```python
from build123d import *

# Parameters (mm, degrees)
SM_BASE_FLANGE_1_DEPTH = 90
CUT_EXTRUDE_1_DEPTH    = 10
CUT_EXTRUDE_2_DEPTH    = 10
FILLET_1_R             = 10


# Sheet-metal steps are written as plain solids
with BuildPart() as part:
    # Sketch 1 → 基体-法兰1 (new body)
    with BuildSketch(Plane.XY):
        with BuildLine():
            Line((0, 0), (34.731899525, 0))
            ThreePointArc((34.731899525, 0), (34.983831563, 0.044422416), (35.205376879, 0.172331663))
            Line((35.205376879, 0.172331663), (57.981333294, 19.283628291))
            Line((57.981333294, 19.283628291), (58.945514708, 18.134561626))
            Line((58.945514708, 18.134561626), (36.169558293, -0.976735001))
            ThreePointArc((36.169558293, -0.976735001), (35.496861778, -1.365116516), (34.731899525, -1.5))
            Line((34.731899525, -1.5), (0, -1.5))
            Line((0, -1.5), (0, 0))
        make_face()
    extrude(amount=SM_BASE_FLANGE_1_DEPTH)

    # 草图6 → 切除-拉伸1 (cut)
    with BuildSketch(Plane(origin=(0, 0, 0), x_dir=(1, 0, 0), z_dir=(0, 1, 0))):
        with BuildLine():
            Line((11, -12.5), (11, -77.5))
            ThreePointArc((11, -77.5), (9, -79.5), (7, -77.5))
            Line((7, -77.5), (7, -12.5))
            ThreePointArc((7, -12.5), (9, -10.5), (11, -12.5))
        make_face()
        with BuildLine():
            Line((26, -12.5), (26, -77.5))
            ThreePointArc((26, -77.5), (24, -79.5), (22, -77.5))
            Line((22, -77.5), (22, -12.5))
            ThreePointArc((22, -12.5), (24, -10.5), (26, -12.5))
        make_face()
    extrude(amount=-CUT_EXTRUDE_1_DEPTH, mode=Mode.SUBTRACT)

    # 草图7 → 切除-拉伸2 (cut)
    with BuildSketch(Plane(origin=(14.461156891, -17.234135678, 0), x_dir=(0, 0, 1), z_dir=(-0.6427876096865403, 0.7660444431189772, 0))):
        with BuildLine():
            Line((12.5, 46.311555509), (77.5, 46.311555509))
            ThreePointArc((77.5, 46.311555509), (79.5, 44.311555509), (77.5, 42.311555509))
            Line((77.5, 42.311555509), (12.5, 42.311555509))
            ThreePointArc((12.5, 42.311555509), (10.5, 44.311555509), (12.5, 46.311555509))
        make_face()
    extrude(amount=-CUT_EXTRUDE_2_DEPTH, mode=Mode.SUBTRACT)

    # 圆角1
    fillet_1_edges = [part.edges().sort_by_distance(p)[0] for p in [
        (0, -0.75, 90),
        (0, -0.75, 0),
        (58.463424001, 18.709094958, 90),
        (58.463424001, 18.709094958, 0),
    ]]
    fillet(fillet_1_edges, radius=FILLET_1_R)


solid = part.part
```
Check sheet for the modelled part. Datum: model origin and axes. Units: mm. A direction names the side the tool comes from. Coordinates: 2 decimals unless noted, no trailing zeros. Write each loop counter-clockwise with the first axis right and the second up, starting at its lowest first coordinate (ties: lowest second). Pieces come first, ordered by that corner, then holes. Notation, with made-up numbers: (72, -27) -> (129, -27) arc R20 cw to (129, -21) -> close; hole circle Ø10 at (66, 62). An arc over 180 degrees is marked (long way). Use a Markdown table: item, result.
1. Go/stop test with flat-tipped pins: pin 1 Ø5 at (y, z) = (10.5, 32) entering from -X; pin 2 Ø8 at (x, z) = (42.5, 55) entering from +Y; pin 3 Ø4 at (y, z) = (11.5, 48.5) entering from +X. Record where each tip stops, or that it passes through.
Reported:
| item | result |
|---|---|
| pin 1 | stops at x = 44.53 |
| pin 2 | stops at y = 9.65 |
| pin 3 | stops at x = 53.42 |
2. Release check for a two-part mould opening along X. For faces 6 (the flat face through (18, -1.5, 44)), 7 (the cylindrical face through (9, -0.7, 10.5)), 8 (the cylindrical face through (2.85, -0.74, 86.99)) record: pulls with the +X half, pulls with the -X half, needs draft (parallel to the pull), parting line crosses it, or undercut.
Reported:
| item | result |
|---|---|
| face 6 | needs draft |
| face 7 | undercut |
| face 8 | pulls with the -X half |
3. Scan lines: line 1 along Y through (x, z) = (26.5, 36); line 2 along X through (y, z) = (2.25, 72.5); line 3 along Y through (x, z) = (45, 75). Record each from-to range of solid material in increasing order.
Reported:
| item | result |
|---|---|
| line 1 | y = -1.5 to 0 |
| line 2 | x = 37.68 to 40.02 |
| line 3 | y = 6.43 to 8.39 |
4. Sectioned sample at C-C (x = 9). Enter the section's corners in (y, z).
Reported:
| item | result |
|---|---|
| outline | (-1.5, 0.05) -> (0, 0.05) -> (0, 10.5) -> (-1.5, 10.5) -> close; (-1.5, 79.5) -> (0, 79.5) -> (0, 89.95) -> (-1.5, 89.95) -> close |
5. Tool access check on faces 1 (the cylindrical face through (56.167, 16.768, 87.148)), 2 (the cylindrical face through (24, -0.7, 10.5)), 3 (the cylindrical face through (48.9, 10.7, 79.5)), 4 (the cylindrical face through (2.85, -0.74, 3.01)), 5 (the flat face through (17, 0, 44)). Record the directions out of +Z, -Z, +X, -X, +Y, -Y that give a thin tool (end or side, any length) a straight path to the whole face; none if there is none.
Reported:
| item | result |
|---|---|
| face 1 | +Z, +X, +Y |
| face 2 | +Y, -Y |
| face 3 | none |
| face 4 | -Z, -X, +Y, -Y |
| face 5 | +Z, -Z, -X, +Y |
6. Sectioned sample at B-B (x = 24). Enter the section's corners in (y, z).
Reported:
| item | result |
|---|---|
| outline | (-1.5, 0) -> (0, 0) -> (0, 10.5) -> (-1.5, 10.5) -> close; (-1.5, 79.5) -> (0, 79.5) -> (0, 90) -> (-1.5, 90) -> close |
7. Sectioned sample at D-D (x = 32.5). Enter the section's corners in (y, z).
Reported:
| item | result |
|---|---|
| outline | (-1.5, 0) -> (0, 0) -> (0, 90) -> (-1.5, 90) -> close |
8. Sectioned sample at A-A (z = 50.5). Enter the section's corners in (x, y), plus the area to 3 significant figures.
Reported:
| item | result |
|---|---|
| outline | (0, -1.5) -> (7, -1.5) -> (7, 0) -> (0, 0) -> close; (11, -1.5) -> (22, -1.5) -> (22, 0) -> (11, 0) -> close; (26, -1.5) -> (34.73, -1.5) arc R2.24 ccw to (36.17, -0.98) -> (47.84, 8.81) -> (46.87, 9.96) -> (35.21, 0.17) arc R0.74 cw to (34.73, 0) -> (26, 0) -> close; (49.94, 12.53) -> (50.9, 11.39) -> (58.95, 18.13) -> (57.98, 19.28) -> close |
| area | 80.3 mm2 |
